Can you work these out from the model? Positions are in its coordinate system, mm. Give positions to 0.01 mm unless a question says otherwise; leave off trailing zeros. Loops run counter-clockwise (first coordinate to the right, second up) from the corner with the lowest first, then second, coordinate; pieces in that order, holes last. Notation, with made-up numbers: (-19, 35) -> (30, 35) arc R35 ccw to (30, 69) -> close; hole circle Ø6 at (63.5, 20). An arc over 180 degrees is marked (long way). One line per question, with ' | ' between items.
from build123d import *

# Parameters (mm, degrees)
BOSS_EXTRU_1_DEPTH      = 3
ENL_V_MAT_EXTRU_1_REACH = 209.016
ESQUISSE2_W             = 40.2
ESQUISSE2_H             = 20.4
ENL_V_MAT_EXTRU_2_REACH = 209.016
ESQUISSE3_R             = 1.45
CONG_2_R                = 4.7
CONG_3_R                = 10
CONG_5_R                = 2
ENL_V_MAT_EXTRU_3_REACH = 209.016
CONG_6_R                = 1.5
ENL_V_MAT_EXTRU_4_REACH = 209.016
ESQUISSE5_R             = 1.15
ESQUISSE6_R             = 1.15
ENL_V_MAT_EXTRU_5_DEPTH = 10


with BuildPart() as part:
    # Esquisse1 → Boss.-Extru.1 (new body)
    with BuildSketch(Plane.XY):
        with BuildLine():
            Line((-30.9, -14), (30.9, -14))
            Line((30.9, -14), (30.9, 14))
            Line((30.9, 14), (-50.9, 14))
            ThreePointArc((-50.9, 14), (-72.161104257, -90.305053327), (-48.1, -194))
            Line((-48.1, -194), (-30.9, -194))
            ThreePointArc((-30.9, -194), (-47.661924206, -104), (-30.9, -14))
        make_face()
    extrude(amount=BOSS_EXTRU_1_DEPTH)

    # Esquisse2 → Enlèv. mat.-Extru.1 (cut, up to next)
    with BuildSketch(Plane.XY.offset(3), mode=Mode.PRIVATE) as enl_v_mat_extru_1_sk1:
        with Locations((1.4, -3.8)):
            Rectangle(ESQUISSE2_W, ESQUISSE2_H)
    enl_v_mat_extru_1_tool1 = extrude(enl_v_mat_extru_1_sk1.sketch, amount=-ENL_V_MAT_EXTRU_1_REACH, mode=Mode.PRIVATE) & part.part
    add(enl_v_mat_extru_1_tool1.solids().sort_by_distance((1.4, -3.8, 3))[0], mode=Mode.SUBTRACT)

    # Esquisse3 → Enlèv. mat.-Extru.2 (cut, up to next)
    with BuildSketch(Plane.XY.offset(3), mode=Mode.PRIVATE) as enl_v_mat_extru_2_sk1:
        with Locations((26.2, -8.8)):
            Circle(ESQUISSE3_R)
    enl_v_mat_extru_2_tool1 = extrude(enl_v_mat_extru_2_sk1.sketch, amount=-ENL_V_MAT_EXTRU_2_REACH, mode=Mode.PRIVATE) & part.part
    # Esquisse3 → Enlèv. mat.-Extru.2 (cut, up to next)
    with BuildSketch(Plane.XY.offset(3), mode=Mode.PRIVATE) as enl_v_mat_extru_2_sk2:
        with Locations((-23.4, -8.8)):
            Circle(ESQUISSE3_R)
    enl_v_mat_extru_2_tool2 = extrude(enl_v_mat_extru_2_sk2.sketch, amount=-ENL_V_MAT_EXTRU_2_REACH, mode=Mode.PRIVATE) & part.part
    # Esquisse3 → Enlèv. mat.-Extru.2 (cut, up to next)
    with BuildSketch(Plane.XY.offset(3), mode=Mode.PRIVATE) as enl_v_mat_extru_2_sk3:
        with Locations((-23.4, 1.2)):
            Circle(ESQUISSE3_R)
    enl_v_mat_extru_2_tool3 = extrude(enl_v_mat_extru_2_sk3.sketch, amount=-ENL_V_MAT_EXTRU_2_REACH, mode=Mode.PRIVATE) & part.part
    # Esquisse3 → Enlèv. mat.-Extru.2 (cut, up to next)
    with BuildSketch(Plane.XY.offset(3), mode=Mode.PRIVATE) as enl_v_mat_extru_2_sk4:
        with Locations((26.2, 1.2)):
            Circle(ESQUISSE3_R)
    enl_v_mat_extru_2_tool4 = extrude(enl_v_mat_extru_2_sk4.sketch, amount=-ENL_V_MAT_EXTRU_2_REACH, mode=Mode.PRIVATE) & part.part
    add(enl_v_mat_extru_2_tool1.solids().sort_by_distance((26.2, -8.8, 3))[0], mode=Mode.SUBTRACT)
    add(enl_v_mat_extru_2_tool2.solids().sort_by_distance((-23.4, -8.8, 3))[0], mode=Mode.SUBTRACT)
    add(enl_v_mat_extru_2_tool3.solids().sort_by_distance((-23.4, 1.2, 3))[0], mode=Mode.SUBTRACT)
    add(enl_v_mat_extru_2_tool4.solids().sort_by_distance((26.2, 1.2, 3))[0], mode=Mode.SUBTRACT)

    # Congé2
    cong_2_edges = [part.edges().sort_by_distance(p)[0] for p in [
        (30.9, -14, 1.5),
        (30.9, 14, 1.5),
    ]]
    fillet(cong_2_edges, radius=CONG_2_R)

    # Congé3
    cong_3_edges = [part.edges().sort_by_distance(p)[0] for p in [
        (-30.9, -14, 1.5),
        (-50.9, 14, 1.5),
    ]]
    fillet(cong_3_edges, radius=CONG_3_R)

    # Congé5
    cong_5_edges = [part.edges().sort_by_distance(p)[0] for p in [
        (-30.9, -194, 1.5),
        (-48.1, -194, 1.5),
    ]]
    fillet(cong_5_edges, radius=CONG_5_R)

    # Esquisse4 → Enlèv. mat.-Extru.3 (cut, up to next)
    with BuildSketch(Plane.XY.offset(3), mode=Mode.PRIVATE) as enl_v_mat_extru_3_sk1:
        Polygon((-33.536552076, -11.101012911), (-42.351911307, -30.013593499), (-48.987474587, -1.620621605), align=None)
    enl_v_mat_extru_3_tool1 = extrude(enl_v_mat_extru_3_sk1.sketch, amount=-ENL_V_MAT_EXTRU_3_REACH, mode=Mode.PRIVATE) & part.part
    # Esquisse4 → Enlèv. mat.-Extru.3 (cut, up to next)
    with BuildSketch(Plane.XY.offset(3), mode=Mode.PRIVATE) as enl_v_mat_extru_3_sk2:
        Polygon((-52.917399073, -8.972975376), (-47.213856869, -33.377913835), (-62.359919338, -49.92921121), align=None)
    enl_v_mat_extru_3_tool2 = extrude(enl_v_mat_extru_3_sk2.sketch, amount=-ENL_V_MAT_EXTRU_3_REACH, mode=Mode.PRIVATE) & part.part
    # Esquisse4 → Enlèv. mat.-Extru.3 (cut, up to next)
    with BuildSketch(Plane.XY.offset(3), mode=Mode.PRIVATE) as enl_v_mat_extru_3_sk3:
        Polygon((-43.711860923, -37.698000672), (-64.383676275, -60.287724165), (-65.97140029, -93.194177891), align=None)
    enl_v_mat_extru_3_tool3 = extrude(enl_v_mat_extru_3_sk3.sketch, amount=-ENL_V_MAT_EXTRU_3_REACH, mode=Mode.PRIVATE) & part.part
    # Esquisse4 → Enlèv. mat.-Extru.3 (cut, up to next)
    with BuildSketch(Plane.XY.offset(3), mode=Mode.PRIVATE) as enl_v_mat_extru_3_sk4:
        Polygon((-46.457316631, 3.078230456), (-30.351945171, -6.80371824), (-30.351945171, 9.155359803), align=None)
    enl_v_mat_extru_3_tool4 = extrude(enl_v_mat_extru_3_sk4.sketch, amount=-ENL_V_MAT_EXTRU_3_REACH, mode=Mode.PRIVATE) & part.part
    # Esquisse4 → Enlèv. mat.-Extru.3 (cut, up to next)
    with BuildSketch(Plane.XY.offset(3), mode=Mode.PRIVATE) as enl_v_mat_extru_3_sk5:
        Polygon((-52.234282619, -74.177445722), (-65.087399313, -106.222081959), (-56.206990273, -139.61663464), align=None)
    enl_v_mat_extru_3_tool5 = extrude(enl_v_mat_extru_3_sk5.sketch, amount=-ENL_V_MAT_EXTRU_3_REACH, mode=Mode.PRIVATE) & part.part
    add(enl_v_mat_extru_3_tool1.solids().sort_by_distance((-41.625313, -14.245076, 3))[0], mode=Mode.SUBTRACT)
    add(enl_v_mat_extru_3_tool2.solids().sort_by_distance((-54.163725, -30.760033, 3))[0], mode=Mode.SUBTRACT)
    add(enl_v_mat_extru_3_tool3.solids().sort_by_distance((-58.022312, -63.726634, 3))[0], mode=Mode.SUBTRACT)
    add(enl_v_mat_extru_3_tool4.solids().sort_by_distance((-35.720402, 1.809957, 3))[0], mode=Mode.SUBTRACT)
    add(enl_v_mat_extru_3_tool5.solids().sort_by_distance((-57.842891, -106.672054, 3))[0], mode=Mode.SUBTRACT)

    # Congé6
    cong_6_edges = [part.edges().sort_by_distance(p)[0] for p in [
        (-62.359919338, -49.92921121, 1.5),
        (-52.917399073, -8.972975376, 1.5),
        (-47.213856869, -33.377913835, 1.5),
        (-46.457316631, 3.078230456, 1.5),
        (-30.351945171, 9.155359803, 1.5),
        (-30.351945171, -6.80371824, 1.5),
        (-52.234282619, -74.177445722, 1.5),
        (-56.206990273, -139.61663464, 1.5),
        (-65.087399313, -106.222081959, 1.5),
        (-43.711860923, -37.698000672, 1.5),
        (-65.97140029, -93.194177891, 1.5),
        (-64.383676275, -60.287724165, 1.5),
        (-48.987474587, -1.620621605, 1.5),
        (-33.536552076, -11.101012911, 1.5),
        (-42.351911307, -30.013593499, 1.5),
    ]]
    fillet(cong_6_edges, radius=CONG_6_R)

    # Esquisse5 → Enlèv. mat.-Extru.4 (cut, up to next)
    with BuildSketch(Plane.XY.offset(3), mode=Mode.PRIVATE) as enl_v_mat_extru_4_sk1:
        with Locations((16.4, 8.9)):
            Circle(ESQUISSE5_R)
    enl_v_mat_extru_4_tool1 = extrude(enl_v_mat_extru_4_sk1.sketch, amount=-ENL_V_MAT_EXTRU_4_REACH, mode=Mode.PRIVATE) & part.part
    # Esquisse5 → Enlèv. mat.-Extru.4 (cut, up to next)
    with BuildSketch(Plane.XY.offset(3), mode=Mode.PRIVATE) as enl_v_mat_extru_4_sk2:
        with Locations((6.4, 8.9)):
            Circle(ESQUISSE5_R)
    enl_v_mat_extru_4_tool2 = extrude(enl_v_mat_extru_4_sk2.sketch, amount=-ENL_V_MAT_EXTRU_4_REACH, mode=Mode.PRIVATE) & part.part
    add(enl_v_mat_extru_4_tool1.solids().sort_by_distance((16.4, 8.9, 3))[0], mode=Mode.SUBTRACT)
    add(enl_v_mat_extru_4_tool2.solids().sort_by_distance((6.4, 8.9, 3))[0], mode=Mode.SUBTRACT)

    # Esquisse6 → Enlèv. mat.-Extru.5 (cut)
    with BuildSketch(Plane.XY.offset(3)):
        with Locations((-45.64268297, -191.5)):
            Circle(ESQUISSE6_R)
        with Locations((-35.64268297, -191.5)):
            Circle(ESQUISSE6_R)
    extrude(amount=-ENL_V_MAT_EXTRU_5_DEPTH, mode=Mode.SUBTRACT)


solid = part.part
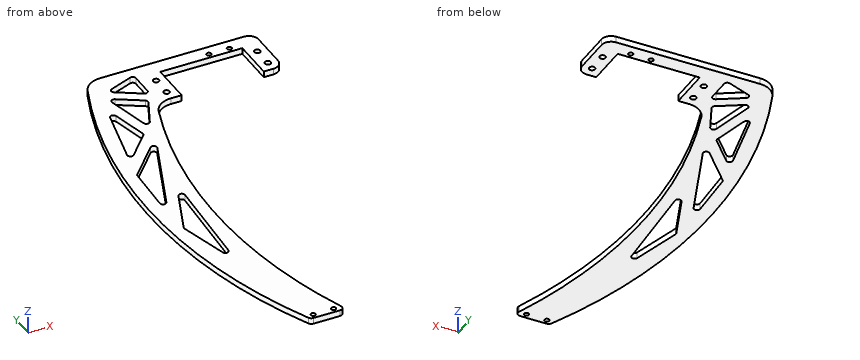
Q1. For pin 1 Ø1.5 at (x, z) = (-48.5, 0.5) entering from -Y; pin 2 Ø1 at (y, z) = (-45, 1.5) entering from +X; pin 3 Ø0.9 at (x, z) = (-8.5, 1.5) entering from -Y, each with a flat end and sliding along its axis, tell me the tip position at first contact or that it passes through.
Entries:
pin 1: y = -193.78 | pin 2: x = -40.48 | pin 3: y = 6.4
Q2. If we section it at B-B (z = 1.2): State how many separate pieces and enclosed holes the cut face has, plus the area to 3 significant figures.
Entries:
separate pieces: 1 | enclosed holes: 13 | area: 4,710 mm²
Q3. If I drill on probe 1 along Y at (x, z) = (26.2, 2.45); probe 2 along Y at (x, z) = (16.4, 1.1); probe 3 along X at (y, z) = (-25, 2.15), over which ranges is the centre line in solid material (lowest first)? Write a range as from..to.
Entries:
probe 1: -14..-10.25, -7.35..-0.25, 2.65..14 | probe 2: 6.4..7.75, 10.05..14 | probe 3: -64.39..-56.61, -49.17..-43.52, -40.02..-34.85
Q4. If we section it at A-A (y = -66): Write out the boundary of the cut face in (x, z).
Entries:
outline: (-71.31, 0) -> (-64.66, 0) -> (-64.66, 3) -> (-71.31, 3) -> close; (-55.06, 0) -> (-44.76, 0) -> (-44.76, 3) -> (-55.06, 3) -> close
